```python
from build123d import *

# Parameters (mm, degrees)
F0_R     = 4
F1_DEPTH = 25


with BuildPart() as f1:
    # F0 (on Top) → F1 (new body)
    with BuildSketch(Plane.XY):
        with BuildLine():
            ThreePointArc((-35, -104.5), (-33.535534, -108.035534), (-30, -109.5))
            Line((-30, -109.5), (30, -109.5))
            ThreePointArc((30, -109.5), (33.535534, -108.035534), (35, -104.5))
            Line((35, -104.5), (35, 104.5))
            ThreePointArc((35, 104.5), (33.535534, 108.035534), (30, 109.5))
            Line((30, 109.5), (-30, 109.5))
            ThreePointArc((-30, 109.5), (-33.535534, 108.035534), (-35, 104.5))
            Line((-35, 104.5), (-35, -104.5))
        make_face()
        with Locations((-17, -90.5)):
            Circle(F0_R, mode=Mode.SUBTRACT)
        with Locations((-17, 0.5)):
            Circle(F0_R, mode=Mode.SUBTRACT)
        with BuildLine():
            ThreePointArc((-30.5, 62.75), (-21.75, 71.5), (-13, 62.75))
            Line((-13, 62.75), (-13, 49.25))
            ThreePointArc((-13, 49.25), (-21.75, 40.5), (-30.5, 49.25))
            Line((-30.5, 49.25), (-30.5, 62.75))
        make_face(mode=Mode.SUBTRACT)
    extrude(amount=F1_DEPTH)


solid = f1.part
```
Work out the finished part from the listing and answer in its coordinate system (mm). A direction names the side the tool comes from. Give positions to 0.01 mm unless a question says otherwise; leave off trailing zeros. Write each loop counter-clockwise with the first axis right and the second up, starting at its lowest first coordinate (ties: lowest second). Pieces come first, ordered by that corner, then holes. Notation, with made-up numbers: (13, -3) - (56, -3) arc R17 ccw to (56, 18) - close; hole circle Ø2 at (16, 35.5). An arc over 180 degrees is marked (long way). Use one line per item in the form item = value.
1. For faces 1 (the face through (-13, 56, 12)), 2 (the face through (0, 2, 25)), determine the directions among +Z, -Z, +X, -X, +Y, -Y from which every point of the face is accessible in a straight line to the end or side of a thin tool.
Filled in:
face_1 = +Z, -Z
face_2 = +Z, +X, -X, +Y, -Y
2. Consider L1, parallel to X at y = 56.5, z = 11; L2, parallel to Y at x = -17, z = 13.25; L3, parallel to Y at x = -15.5, z = 16. Determine where each line is inside the solid, lowest interval first.
Filled in:
L1 = -35 to -30.5, -13 to 35
L2 = -109.5 to -94.5, -86.5 to -3.5, 4.5 to 41.9, 70.1 to 109.5
L3 = -109.5 to -94.21, -86.79 to -3.21, 4.21 to 43.13, 68.87 to 109.5
3. A cutting plane is placed at B-B (x = -15.5). Write down the section's boundary in (y, z), and give its area (3 significant figures).
Filled in:
outline = (-109.5, 0) - (-94.21, 0) - (-94.21, 25) - (-109.5, 25) - close; (-86.79, 0) - (-3.21, 0) - (-3.21, 25) - (-86.79, 25) - close; (4.21, 0) - (43.13, 0) - (43.13, 25) - (4.21, 25) - close; (68.87, 0) - (109.5, 0) - (109.5, 25) - (68.87, 25) - close
area = 4,460 mm^2
4. A cutting plane is placed at C-C (z = 16.5). Write down the section's boundary in (x, y).
Filled in:
outline = (-35, -104.5) arc R5 ccw to (-30, -109.5) - (30, -109.5) arc R5 ccw to (35, -104.5) - (35, 104.5) arc R5 ccw to (30, 109.5) - (-30, 109.5) arc R5 ccw to (-35, 104.5) - close; hole (-30.5, 49.25) arc R8.75 ccw to (-13, 49.25) - (-13, 62.75) arc R8.75 ccw to (-30.5, 62.75) - close; hole circle Ø8 at (-17, -90.5); hole circle Ø8 at (-17, 0.5)
5. Determine the mould class of faces 3 (the face through (-35, 1, 12)), 4 (the face through (33.5, -108.07, 12.32)), 5 (the face through (-17.867, -94.405, 12.325)) for opening direction Y: released by +Y, released by -Y, zero draft, split by the parting line, or undercut.
Filled in:
face_3 = zero draft
face_4 = released by -Y
face_5 = undercut
6. A cutting plane is placed at A-A (y = -90.5). Write down the section's boundary in (x, z).
Filled in:
outline = (-35, 0) - (-21, 0) - (-21, 25) - (-35, 25) - close; (-13, 0) - (35, 0) - (35, 25) - (-13, 25) - close
